from build123d import *

# Parameters (mm, degrees)
SKETCH_1_W          = 10
SKETCH_1_H          = 10
EXTRUDE_1_DEPTH     = 10
SKETCH_3_R          = 1.6
CUT_EXTRUDE_1_DEPTH = 32


with BuildPart() as part:
    # Эскиз1 → Бобышка-Вытянуть1 (new body)
    with BuildSketch(Plane.XY):
        with Locations((-25, 11)):
            Rectangle(SKETCH_1_W, SKETCH_1_H)
        with BuildLine():
            ThreePointArc((12.560254774, -16), (0, -4.4), (-12.560254774, -16))
            Line((-12.560254774, -16), (-20, -16))
            Line((-20, -16), (-20, 16))
            Line((-20, 16), (20, 16))
            Line((20, 16), (20, -16))
            Line((20, -16), (12.560254774, -16))
        make_face()
        with Locations((-25, -11)):
            Rectangle(SKETCH_1_W, SKETCH_1_H)
        with Locations((25, 11)):
            Rectangle(SKETCH_1_W, SKETCH_1_H)
        with Locations((25, -11)):
            Rectangle(SKETCH_1_W, SKETCH_1_H)
    extrude(amount=EXTRUDE_1_DEPTH)

    # Эскиз3 → Вырез-Вытянуть1 (cut)
    with BuildSketch(Plane(origin=(0, 16, 0), x_dir=(1, 0, 0), z_dir=(0, 1, 0))):
        with Locations(Location((-25, -5, 0), (0, 0, 270))):
            Circle(SKETCH_3_R)
        with Locations(Location((25, -5, 0), (0, 0, 180))):
            Circle(SKETCH_3_R)
    extrude(amount=-CUT_EXTRUDE_1_DEPTH, mode=Mode.SUBTRACT)


solid = part.part
The listing builds one solid part. Answer for the finished solid, in the listing's coordinates (mm). A direction names the side the tool comes from. Give positions to 0.01 mm unless a question says otherwise; leave off trailing zeros. Write each loop counter-clockwise with the first axis right and the second up, starting at its lowest first coordinate (ties: lowest second). Pieces come first, ordered by that corner, then holes. Notation, with made-up numbers: (-30.5, 23.5) - (-20.5, 23.5) arc R4 cw to (-20.5, 27.5) - close; hole circle Ø2 at (-18, 36). An arc over 180 degrees is marked (long way). Use a Markdown table: item, result.
1. Section D-D on z = 1 is taken. Write down the section's boundary in (x, y).
Values follow:
| item | result |
|---|---|
| outline | (-30, -16) - (-12.56, -16) arc R12.6 cw to (12.56, -16) - (30, -16) - (30, -6) - (20, -6) - (20, 6) - (30, 6) - (30, 16) - (-30, 16) - (-30, 6) - (-20, 6) - (-20, -6) - (-30, -6) - close |
2. Each of these flat-tipped pins is pushed along its axis until it touches: P1, Ø5, axis at x = -2, y = 2.5, coming from the -Z side; P2, Ø5, axis at y = -1.5, z = 2.5, coming from the -X side. Where does it stop, or does it pass through?
Values follow:
| item | result |
|---|---|
| P1 | stops at z = 0 |
| P2 | stops at x = -20 |
3. Section B-B on z = 5 is taken. Count the separate pieces of the cut face and the enclosed holes in it, plus the area to 3 significant figures.
Values follow:
| item | result |
|---|---|
| separate pieces | 5 |
| enclosed holes | 0 |
| area | 1,330 mm² |
4. A tool of negligible diameter and unlimited length cuts with its end or side. For faces 4 (the flat face through (-25, -6, 3)), 5 (the flat face through (23, -6, 5)), 6 (the flat face through (30, -11, 5)), from which of +Z, -Z, +X, -X, +Y, -Y can it reach the whole face along a straight path? Write none if from no direction.
Values follow:
| item | result |
|---|---|
| face 4 | +Z, -Z, -X |
| face 5 | +Z, -Z, +X |
| face 6 | +Z, -Z, +X, +Y, -Y |
5. Section A-A on x = 25 is taken. Write down the section's boundary in (y, z), plus the area to 3 significant figures.
Values follow:
| item | result |
|---|---|
| outline | (-16, 0) - (-6, 0) - (-6, 3.4) - (-16, 3.4) - close; (-16, 6.6) - (-6, 6.6) - (-6, 10) - (-16, 10) - close; (6, 0) - (16, 0) - (16, 3.4) - (6, 3.4) - close; (6, 6.6) - (16, 6.6) - (16, 10) - (6, 10) - close |
| area | 136 mm² |
6. Find the intervals of material crossed by probe 1 along Y at (x, z) = (21, 6); probe 2 along Z at (x, y) = (25, 10); probe 3 along X at (y, z) = (-12, 6.25), in increasing order. Write a range as from..to.
Values follow:
| item | result |
|---|---|
| probe 1 | y = -16..-6, 6..16 |
| probe 2 | z = 0..3.4, 6.6..10 |
| probe 3 | x = -30..-26, -24..-11.57, 11.57..24, 26..30 |
7. For a pull along Z with two mould halves and no side action, classify faces 1 (the cylindrical face through (-23.414, 11.07, 4.792)), 2 (the flat face through (0, 0, 10)), 3 (the flat face through (21, -16, 5)) as released by +Z, released by -Z, zero draft, split by the parting line, or undercut.
Values follow:
| item | result |
|---|---|
| face 1 | undercut |
| face 2 | released by +Z |
| face 3 | zero draft |
8. Section C-C on y = 9 is taken. Write down the section's boundary in (x, z), plus the area to 3 significant figures.
Values follow:
| item | result |
|---|---|
| outline | (-30, 0) - (30, 0) - (30, 10) - (-30, 10) - close; hole circle Ø3.2 at (-25, 5); hole circle Ø3.2 at (25, 5) |
| area | 584 mm² |
